Source: CAD feature listing. Evaluate the final solid. Frame: model axes, mm. Coordinates: 2 decimals unless noted, no trailing zeros. Order: outer loops, then holes, each group sorted by start corner. A loop starts at its lowest first (then second) coordinate and runs counter-clockwise, first axis right, second up. Notation, with made-up numbers: (-9, 20) -> (6, 20) arc R14 cw to (6, 27) -> close; hole circle Ø9 at (85.25, 0.5). An arc over 180 degrees is marked (long way). Put each result on its own line as item: value.
Autodesk Inventor part; units mm, degrees
ref_plane "YZ Plane" through (0, 0, 0) normal (1, 0, 0) x (0, 1, 0)
ref_plane "XZ Plane" through (0, 0, 0) normal (0, 1, 0) x (-1, 0, 0)
ref_plane "XY Plane" through (0, 0, 0) normal (0, 0, 1) x (1, 0, 0)
sketch "Эскиз1" plane through (0, 0, 0) normal (0, 0, 1) x (1, 0, 0)
  circle A0 centre (0, 0) radius 10
  dimension "d0" = 20
extrude "Выдавливание1" add sketch "Эскиз1" along normal blind 100
sketch "Эскиз2" plane through (0, 0, 100) normal (0, 0, 1) x (1, 0, 0)
  circle A0 centre (0, 0) radius 10
  line L0 (8, 6) -> (-8, 6)
  line L1 (-8, -6) -> (8, -6)
  dimension "d3" = 12
extrude "Выдавливание2" cut sketch "Эскиз2" against normal blind 6 contours L0 A0 | A0 L1
equation "\"d0\" = d_main_shaft"
equation "\"d3\" = width_flattened_surface"
equation "\"d4\" = 2 * thickness_steel"
equation "\"d_main_shaft\" = 20"
equation "\"tolerance_plazma\" = 0.1"
equation "\"thickness_steel\" = 3"
equation "\"d_main_screw_holes\" = 6.1"
equation "\"thickness_profile_tibea\" = 3"
equation "\"thickness_profile_femur\" = 3"
equation "\"width_flattened_surface\" = 12"
equation "\"width_shaft_shift\" = 35"
equation "\"hight_shaft_shift\" = 37"
properties part number "shaft_tibea" material "Сталь"
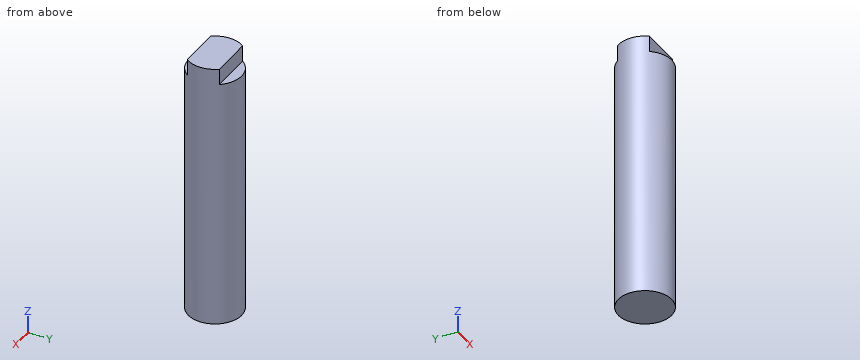
1. Cut plane B-B on z = 88.5. Output: boundary loops of the cut face in (x, y).
Numbers:
outline: circle Ø20 at (0, 0)
2. Cut plane A-A on x = 0. Output: boundary loops of the cut face in (y, z).
Numbers:
outline: (-10, 0) -> (10, 0) -> (10, 94) -> (6, 94) -> (6, 100) -> (-6, 100) -> (-6, 94) -> (-10, 94) -> close
3. Ray query, line 1 along Y through (x, z) = (-0.5, 78.5); line 2 along X through (y, z) = (-8, 53); line 3 along X through (y, z) = (6, 86). Return the intervals inside material, ascending.
Numbers:
line 1: y = -9.99 to 9.99
line 2: x = -6 to 6
line 3: x = -8 to 8
4. First-contact query: pin 1 (1.2 mm diameter, centred on x = -4, y = 8.5, fed in from +Z); pin 2 (2 mm diameter, centred on y = -5, z = 49, fed in from -X); pin 3 (5 mm diameter, centred on x = 5.5, z = 52, fed in from +Y). Flat tips, straight axial feed; report the tip coordinate or a pass-through.
Numbers:
pin 1: stops at z = 94
pin 2: stops at x = -9.17
pin 3: stops at y = 9.54
5. Cut plane C-C on y = 7.75. Output: boundary loops of the cut face in (x, z).
Numbers:
outline: (-6.32, 0) -> (6.32, 0) -> (6.32, 94) -> (-6.32, 94) -> close
6. Cut plane D-D on x = -6.75. Output: boundary loops of the cut face in (y, z).
Numbers:
outline: (-7.38, 0) -> (7.38, 0) -> (7.38, 94) -> (6, 94) -> (6, 100) -> (-6, 100) -> (-6, 94) -> (-7.38, 94) -> close
